Part print with two shaded views. Sizes in mm from the minimum x, y, z corner. A direction names the side the tool comes from. Round coordinates to 2 decimals unless told otherwise and drop trailing zeros. Loops run counter-clockwise (first coordinate to the right, second up) from the corner with the lowest first, then second, coordinate; pieces in that order, holes last. Notation, with made-up numbers: M 54.25,-2 L 110.25,-2 A17 ccw 110.25,21 Z; hole C 61,-36 d9. An arc over 180 degrees is marked long. Answer as CSV lines item,"result". Start each with the question number.
Item 1: Drop flat-ended pins along their axis: pin 1 Ø3 at (x, y) = (123, 2) entering from +Z; pin 2 Ø12 at (x, y) = (141, 182.5) entering from +Z. Give the stop position or say it passes through.
Item 2: Band-saw the part on A-A (z = 99.5). Give the cut face in (x, y).
Item 3: Band-saw the part on B-B (x = 95). Give the cut face in (y, z).
Item 4: Mould opens along Y. For the marked faces 1, 2, 3 and 4 say: pulls with the +Y half, pulls with the -Y half, needs draft (parallel to the pull), parting line crosses it, or undercut.
Item 5: Wall check: line 1 (Y direction, x = 34.5, z = 50); line 2 (X direction, y = 78, z = 53); line 3 (Z direction, x = 258.5, y = 77). Give the ranges that are in metal, low to high.
Item 6: Which spindle directions (+Z, -Z, +X, -X, +Y, -Y) get a long thin tool onto all of the face, cutting with end or side? Do the marked faces 5 and 6. Say none if no direction does.
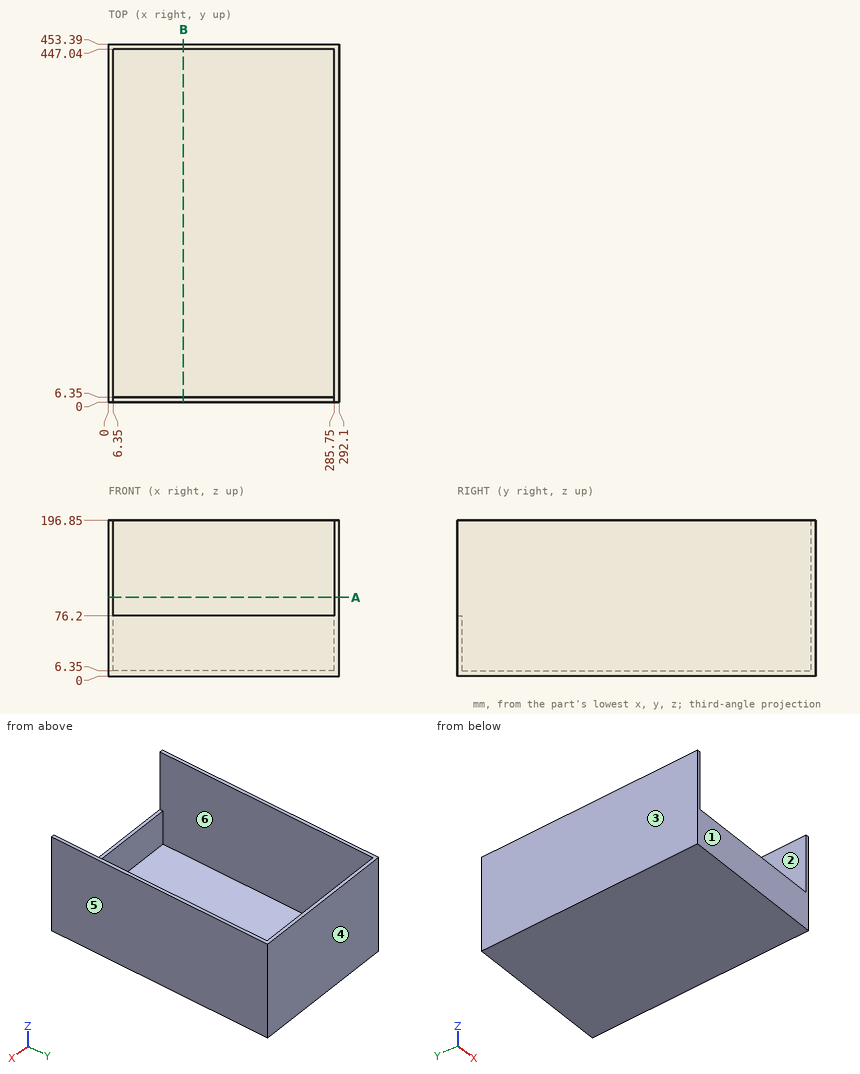
Answer block:
1,pin 1,"stops at z = 76.2"
1,pin 2,"stops at z = 6.35"
2,outline,"M 0,0 L 6.35,0 L 6.35,447.04 L 285.75,447.04 L 285.75,0 L 292.1,0 L 292.1,453.39 L 0,453.39 Z"
3,outline,"M 0,0 L 453.39,0 L 453.39,196.85 L 447.04,196.85 L 447.04,6.35 L 6.35,6.35 L 6.35,76.2 L 0,76.2 Z"
4,face 1,"pulls with the -Y half"
4,face 2,"undercut"
4,face 3,"needs draft"
4,face 4,"pulls with the +Y half"
5,line 1,"y = 0 to 6.35, 447.04 to 453.39"
5,line 2,"x = 0 to 6.35, 285.75 to 292.1"
5,line 3,"z = 0 to 6.35"
6,face 5,"+Z, -Z, +X, +Y, -Y"
6,face 6,"+Z"
